Geometry check sheet. Reference: the model listing, model coordinates, mm. Round coordinates to 2 decimals unless told otherwise and drop trailing zeros. Write each loop counter-clockwise with the first axis right and the second up, starting at its lowest first coordinate (ties: lowest second). Pieces come first, ordered by that corner, then holes.
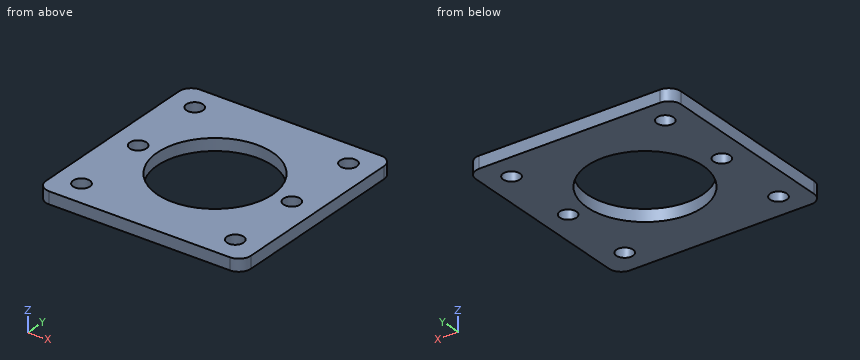
from build123d import *

# Parameters (mm, degrees)
SKETCH1_W           = 50.8
SKETCH1_H           = 50.8
SKETCH1_R           = 14.2875
SKETCH1_R_2         = 2.07
BOSS_EXTRUDE1_DEPTH = 1.5
FILLET1_R           = 3


with BuildPart() as part:
    # Sketch1 → Boss-Extrude1 (new, symmetric)
    with BuildSketch(Plane.XY):
        Rectangle(SKETCH1_W, SKETCH1_H)
        Circle(SKETCH1_R, mode=Mode.SUBTRACT)
        with Locations((-19.05, 19.05)):
            Circle(SKETCH1_R_2, mode=Mode.SUBTRACT)
        with Locations(Location((19.05, -19.05, 0), (0, 0, 180))):
            Circle(SKETCH1_R_2, mode=Mode.SUBTRACT)
        with Locations((19.05, 19.05)):
            Circle(SKETCH1_R_2, mode=Mode.SUBTRACT)
        with Locations((-19.05, -19.05)):
            Circle(SKETCH1_R_2, mode=Mode.SUBTRACT)
        with Locations((-19.05, 0)):
            Circle(SKETCH1_R_2, mode=Mode.SUBTRACT)
        with Locations(Location((19.05, 0, 0), (0, 0, 180))):
            Circle(SKETCH1_R_2, mode=Mode.SUBTRACT)
    extrude(amount=BOSS_EXTRUDE1_DEPTH, both=True)

    # Fillet1
    fillet1_edges = [part.edges().sort_by_distance(p)[0] for p in [
        (25.4, -25.4, 0),
        (-25.4, -25.4, 0),
        (-25.4, 25.4, 0),
        (25.4, 25.4, 0),
    ]]
    fillet(fillet1_edges, radius=FILLET1_R)


solid = part.part
1. Section check C-C (z = 0.7). State how many separate pieces and enclosed holes the cut face has, plus the area to 3 significant figures.
2. Section check D-D (x = 0). Record the cut outline in (y, z).
3. Section check B-B (x = -19.05). Record the cut outline in (y, z).
4. Scan lines: line 1 along X through (y, z) = (-19, 0.35); line 2 along Y through (x, z) = (-19.05, -0.05); line 3 along Y through (x, z) = (-0.5, -1.05). Record each from-to range of solid material in increasing order.
5. Section check A-A (y = -19.05). Record the cut outline in (x, z), plus the area to 3 significant figures.
6. Depth check by flat-ended pin: pin 1 Ø2.5 at (x, y) = (19.05, -19.05) entering from -Z. Enter the tip coordinate at first touch or a pass-through.
Results below:
1. separate pieces: 1
1. enclosed holes: 7
1. area: 1,850 mm2
2. outline: (-25.4, -1.5) - (-14.29, -1.5) - (-14.29, 1.5) - (-25.4, 1.5) - close; (14.29, -1.5) - (25.4, -1.5) - (25.4, 1.5) - (14.29, 1.5) - close
3. outline: (-25.4, -1.5) - (-21.12, -1.5) - (-21.12, 1.5) - (-25.4, 1.5) - close; (-16.98, -1.5) - (-2.07, -1.5) - (-2.07, 1.5) - (-16.98, 1.5) - close; (2.07, -1.5) - (16.98, -1.5) - (16.98, 1.5) - (2.07, 1.5) - close; (21.12, -1.5) - (25.4, -1.5) - (25.4, 1.5) - (21.12, 1.5) - close
4. line 1: x = -25.4 to -21.12, -16.98 to 16.98, 21.12 to 25.4
4. line 2: y = -25.4 to -21.12, -16.98 to -2.07, 2.07 to 16.98, 21.12 to 25.4
4. line 3: y = -25.4 to -14.28, 14.28 to 25.4
5. outline: (-25.4, -1.5) - (-21.12, -1.5) - (-21.12, 1.5) - (-25.4, 1.5) - close; (-16.98, -1.5) - (16.98, -1.5) - (16.98, 1.5) - (-16.98, 1.5) - close; (21.12, -1.5) - (25.4, -1.5) - (25.4, 1.5) - (21.12, 1.5) - close
5. area: 128 mm2
6. pin 1: passes through
